Check sheet for the modelled part. Datum: model origin and axes. Units: mm. Give positions to 0.01 mm unless a question says otherwise; leave off trailing zeros. Order: outer loops, then holes, each group sorted by start corner. A loop starts at its lowest first (then second) coordinate and runs counter-clockwise, first axis right, second up.
from build123d import *

# Parameters (mm, degrees)
SKETCH_1_W          = 0.709981308
SKETCH_1_H          = 0.70422052
EXTRUDE_1_DEPTH     = 10
EXTRUDE_1_2_DEPTH   = 10
EXTRUDE_1_3_DEPTH   = 10
EXTRUDE_1_4_DEPTH   = 10
EXTRUDE_2_DEPTH     = 2.54
SKETCH_4_W          = 10.16
SKETCH_4_H          = 1.54
CUT_EXTRUDE_2_DEPTH = 0.5
SKETCH_1_2_W        = 0.709981308
SKETCH_1_2_H        = 0.70422052
EXTRUDE_3_DEPTH     = 2
CUT_EXTRUDE_1_DEPTH = 2.54
SKETCH_1_3_W        = 0.709981308
SKETCH_1_3_H        = 0.70422052
EXTRUDE_4_DEPTH     = 4.5
CHAMFER_1_SIZE      = 0.1


with BuildPart() as part:
    # Sketch 1 → Extrude 1 (new body)
    with BuildSketch(Plane.XY):
        with Locations((2.54, 0)):
            Rectangle(SKETCH_1_W, SKETCH_1_H)
    extrude(amount=EXTRUDE_1_DEPTH)



with BuildPart() as body_2:
    # Sketch 1 → Extrude 1 2 (new body)
    with BuildSketch(Plane.XY):
        Rectangle(SKETCH_1_W, SKETCH_1_H)
    extrude(amount=EXTRUDE_1_2_DEPTH)


with BuildPart() as body_3:
    # Sketch 1 → Extrude 1 3 (new body)
    with BuildSketch(Plane.XY):
        with Locations((5.08, 0)):
            Rectangle(SKETCH_1_W, SKETCH_1_H)
    extrude(amount=EXTRUDE_1_3_DEPTH)


with BuildPart() as body_4:
    # Sketch 1 → Extrude 1 4 (new body)
    with BuildSketch(Plane.XY):
        with Locations((7.62, 0)):
            Rectangle(SKETCH_1_W, SKETCH_1_H)
    extrude(amount=EXTRUDE_1_4_DEPTH)


with BuildPart() as part_1:
    add(part.part)

    add(body_2.part)  # Extrude 2 merges body 2

    add(body_3.part)  # Extrude 2 merges body 3

    add(body_4.part)  # Extrude 2 merges body 4
    # Sketch 2 → Extrude 2 (add)
    with BuildSketch(Plane.XY):
        Polygon((-1.27, 1.27), (1.27, 1.27), (6.35, 1.27), (8.89, 1.27), (8.89, -1.27), (6.35, -1.27), (1.27, -1.27), (-1.27, -1.27), align=None)
    extrude(amount=EXTRUDE_2_DEPTH)

    # Sketch 4 → Cut-Extrude 2 (cut)
    with BuildSketch(Plane.XY.offset(2.54)):
        with Locations((3.81, 0)):
            Rectangle(SKETCH_4_W, SKETCH_4_H)
    extrude(amount=-CUT_EXTRUDE_2_DEPTH, mode=Mode.SUBTRACT)


with BuildPart() as body_2_2:
    # of the pieces the cut leaves, the one that is kept (cut_extrude_2_keep)
    add(part_1.part.solids().sort_by_distance((8.89, 1.27, 0))[0])

    # Sketch 1_2 → Extrude 3 (add)
    with BuildSketch(Plane.XY):
        with Locations((2.54, 0)):
            Rectangle(SKETCH_1_2_W, SKETCH_1_2_H)
        Rectangle(SKETCH_1_2_W, SKETCH_1_2_H)
        with Locations((5.08, 0)):
            Rectangle(SKETCH_1_2_W, SKETCH_1_2_H)
        with Locations((7.62, 0)):
            Rectangle(SKETCH_1_2_W, SKETCH_1_2_H)
    extrude(amount=-EXTRUDE_3_DEPTH)

    # Sketch 3 → Cut-Extrude 1 (cut)
    with BuildSketch(Plane(origin=(0, 0, 0), x_dir=(-1, 0, 0), z_dir=(0, 0, -1))):
        Polygon((-8.59, 1.27), (-8.89, 0.97), (-8.89, 1.27), align=None)
        Polygon((-6.05, 1.27), (-6.35, 0.97), (-6.65, 1.27), align=None)
        Polygon((-3.51, 1.27), (-3.81, 0.97), (-4.11, 1.27), align=None)
        Polygon((-0.97, 1.27), (-1.27, 0.97), (-1.57, 1.27), align=None)
        Polygon((1.57, 1.27), (1.27, 0.97), (0.97, 1.27), align=None)
        Polygon((0.97, -1.27), (1.57, -1.27), (1.27, -0.97), align=None)
        Polygon((-1.57, -1.27), (-0.97, -1.27), (-1.27, -0.97), align=None)
        Polygon((-4.11, -1.27), (-3.51, -1.27), (-3.81, -0.97), align=None)
        Polygon((-6.65, -1.27), (-6.05, -1.27), (-6.35, -0.97), align=None)
        Polygon((-8.89, -1.27), (-8.89, -0.97), (-8.59, -1.27), align=None)
    extrude(amount=-CUT_EXTRUDE_1_DEPTH, mode=Mode.SUBTRACT)

    # Sketch 1_3 → Extrude 4 (add)
    with BuildSketch(Plane.XY):
        with Locations((2.54, 0)):
            Rectangle(SKETCH_1_3_W, SKETCH_1_3_H)
        Rectangle(SKETCH_1_3_W, SKETCH_1_3_H)
        with Locations((5.08, 0)):
            Rectangle(SKETCH_1_3_W, SKETCH_1_3_H)
        with Locations((7.62, 0)):
            Rectangle(SKETCH_1_3_W, SKETCH_1_3_H)
    extrude(amount=EXTRUDE_4_DEPTH)

    # Chamfer 1
    chamfer_1_edges = [body_2_2.edges().sort_by_distance(p)[0] for p in [
        (0.354990654, 0, -2),
        (0, -0.35211026, -2),
        (-0.354990654, 0, -2),
        (0, 0.35211026, -2),
        (2.894990654, 0, -2),
        (2.54, -0.35211026, -2),
        (2.185009346, 0, -2),
        (2.54, 0.35211026, -2),
        (5.434990654, 0, -2),
        (5.08, -0.35211026, -2),
        (4.725009346, 0, -2),
        (5.08, 0.35211026, -2),
        (7.974990654, 0, -2),
        (7.62, -0.35211026, -2),
        (7.265009346, 0, -2),
        (7.62, 0.35211026, -2),
        (0.354990654, 0, 4.5),
        (0, 0.35211026, 4.5),
        (-0.354990654, 0, 4.5),
        (0, -0.35211026, 4.5),
        (2.894990654, 0, 4.5),
        (2.54, 0.35211026, 4.5),
        (2.185009346, 0, 4.5),
        (2.54, -0.35211026, 4.5),
        (5.434990654, 0, 4.5),
        (5.08, 0.35211026, 4.5),
        (4.725009346, 0, 4.5),
        (5.08, -0.35211026, 4.5),
        (7.974990654, 0, 4.5),
        (7.62, 0.35211026, 4.5),
        (7.265009346, 0, 4.5),
        (7.62, -0.35211026, 4.5),
    ]]
    chamfer(chamfer_1_edges, length=CHAMFER_1_SIZE)


solid = body_2_2.part
1) Section check A-A, the plane y = 1.1. Record the cut outline in (x, z), then the cut area to 3 significant figures.
Recorded:
outline: (-1.14, 0) - (1.14, 0) - (1.14, 2.54) - (-1.14, 2.54) - close; (1.4, 0) - (3.68, 0) - (3.68, 2.54) - (1.4, 2.54) - close; (3.94, 0) - (6.22, 0) - (6.22, 2.54) - (3.94, 2.54) - close; (6.48, 0) - (8.76, 0) - (8.76, 2.54) - (6.48, 2.54) - close
area: 23.2 mm2
2) Draft check along X on faces 1 (the face through (4, 0, 2.04)), 2 (the face through (3, 1.27, 1)), 3 (the face through (8.89, 0, 1)). Enter one of: +X half, -X half, draft (parallel to the pull), parting line (faces both ways), or undercut.
Recorded:
face 1: undercut
face 2: draft
face 3: +X half
3) Material ranges on L1, parallel to X at y = -0.1, z = -1.5 (3 decimals); L2, parallel to Y at x = 5.5, z = 2.25; L3, parallel to Z at x = 5.25, y = 0.85, recorded low to high.
Recorded:
L1: x = -0.355 to 0.355, 2.185 to 2.895, 4.725 to 5.435, 7.265 to 7.975
L2: y = -1.27 to -0.77, 0.77 to 1.27
L3: z = 0 to 2.54
4) Section check C-C, the plane x = 7. Record the cut outline in (y, z), then the cut area to 3 significant figures.
Recorded:
outline: (-1.27, 0) - (1.27, 0) - (1.27, 2.54) - (0.77, 2.54) - (0.77, 2.04) - (-0.77, 2.04) - (-0.77, 2.54) - (-1.27, 2.54) - close
area: 5.68 mm2
5) Section check D-D, the plane z = -0.5. Record the cut outline in (x, y) (3 decimals), then the cut area to 3 significant figures.
Recorded:
outline: (-0.355, -0.352) - (0.355, -0.352) - (0.355, 0.352) - (-0.355, 0.352) - close; (2.185, -0.352) - (2.895, -0.352) - (2.895, 0.352) - (2.185, 0.352) - close; (4.725, -0.352) - (5.435, -0.352) - (5.435, 0.352) - (4.725, 0.352) - close; (7.265, -0.352) - (7.975, -0.352) - (7.975, 0.352) - (7.265, 0.352) - close
area: 2.00 mm2
6) Depth check by flat-ended pin: pin 1 Ø0.8 at (x, z) = (5, -0.5) entering from -Y; pin 2 Ø1.5 at (y, z) = (1, 2) entering from +X; pin 3 Ø0.8 at (y, z) = (0, -1.5) entering from -X (3 decimals). Enter the tip coordinate at first touch or a pass-through.
Recorded:
pin 1: stops at y = -0.35
pin 2: stops at x = 8.89
pin 3: stops at x = -0.355
7) Section check B-B, the plane z = 1.75. Record the cut outline in (x, y).
Recorded:
outline: (-1.27, -0.97) - (-0.97, -1.27) - (0.97, -1.27) - (1.27, -0.97) - (1.57, -1.27) - (3.51, -1.27) - (3.81, -0.97) - (4.11, -1.27) - (6.05, -1.27) - (6.35, -0.97) - (6.65, -1.27) - (8.59, -1.27) - (8.89, -0.97) - (8.89, 0.97) - (8.59, 1.27) - (6.65, 1.27) - (6.35, 0.97) - (6.05, 1.27) - (4.11, 1.27) - (3.81, 0.97) - (3.51, 1.27) - (1.57, 1.27) - (1.27, 0.97) - (0.97, 1.27) - (-0.97, 1.27) - (-1.27, 0.97) - close
